CAD build for the part. Positions are in the model's coordinates, mm. Give positions to 0.01 mm unless a question says otherwise; leave off trailing zeros. Order: outer loops, then holes, each group sorted by start corner. A loop starts at its lowest first (then second) coordinate and runs counter-clockwise, first axis right, second up.
Autodesk Inventor part; units mm, degrees
ref_plane "HW_B_1_XY" through (-30.5, 7, 0) normal (0, 1, 0) x (0, 0, -1)
ref_plane "HW_B_1_YZ" through (-30.5, 7, 0) normal (0, 0, -1) x (-1, 0, 0)
ref_plane "HW_B_1_ZX" through (-30.5, 7, 0) normal (-1, 0, 0) x (0, 1, 0)
sketch "Sketch_1" plane through (0, 0, 0) normal (0, 0, 1) x (0, 1, 0)
  line L0 (3.8889, 0) -> (0, 0)
  arc A0 (0, 26.6) -> (0.6, 26) centre (0.6, 26.6) ccw
  line L1 (0.6, 26) -> (3.2889, 26)
  arc A1 (3.2889, 26) -> (3.8889, 26.6) centre (3.2889, 26.6) ccw
  line L2 (3.8889, 26.6) -> (3.8889, 28.8966)
  arc A2 (3.8889, 32.1034) -> (3.8889, 28.8966) centre (7, 30.5) ccw
  line L3 (3.8889, 32.1034) -> (3.8889, 34.4)
  arc A3 (3.8889, 34.4) -> (3.2889, 35) centre (3.2889, 34.4) ccw
  line L4 (3.2889, 35) -> (0.6, 35)
  arc A4 (0.6, 35) -> (0, 34.4) centre (0.6, 34.4) ccw
  line L5 (0, 34.4) -> (0, 26.6)
revolve "Revolution1" add sketch "Sketch_1" angle 360 about axis through (0, 3.8889, 0) along (0, 1, 0)
ref_plane "HW_B_1_XY" through (-30.5, 7, 0) normal (0, 1, 0) x (0, 0, -1)
ref_plane "HW_B_1_YZ" through (-30.5, 7, 0) normal (0, 0, -1) x (-1, 0, 0)
ref_plane "HW_B_1_ZX" through (-30.5, 7, 0) normal (-1, 0, 0) x (0, 1, 0)
ref_plane "HW_B_10_XY" through (30.5, 7, 0) normal (0, 1, 0) x (0, 0, -1)
ref_plane "HW_B_10_YZ" through (30.5, 7, 0) normal (0, 0, -1) x (-1, 0, 0)
ref_plane "HW_B_10_ZX" through (30.5, 7, 0) normal (-1, 0, 0) x (0, 1, 0)
ref_plane "HW_B_11_XY" through (28.6606, 7, -10.4316) normal (0, 1, 0) x (0, 0, -1)
ref_plane "HW_B_11_YZ" through (28.6606, 7, -10.4316) normal (0, 0, -1) x (-1, 0, 0)
ref_plane "HW_B_11_ZX" through (28.6606, 7, -10.4316) normal (-1, 0, 0) x (0, 1, 0)
ref_plane "HW_B_12_XY" through (23.3644, 7, -19.605) normal (0, 1, 0) x (0, 0, -1)
ref_plane "HW_B_12_YZ" through (23.3644, 7, -19.605) normal (0, 0, -1) x (-1, 0, 0)
ref_plane "HW_B_12_ZX" through (23.3644, 7, -19.605) normal (-1, 0, 0) x (0, 1, 0)
ref_plane "HW_B_13_XY" through (15.25, 7, -26.4138) normal (0, 1, 0) x (0, 0, -1)
ref_plane "HW_B_13_YZ" through (15.25, 7, -26.4138) normal (0, 0, -1) x (-1, 0, 0)
ref_plane "HW_B_13_ZX" through (15.25, 7, -26.4138) normal (-1, 0, 0) x (0, 1, 0)
ref_plane "HW_B_14_XY" through (5.2963, 7, -30.0366) normal (0, 1, 0) x (0, 0, -1)
ref_plane "HW_B_14_YZ" through (5.2963, 7, -30.0366) normal (0, 0, -1) x (-1, 0, 0)
ref_plane "HW_B_14_ZX" through (5.2963, 7, -30.0366) normal (-1, 0, 0) x (0, 1, 0)
ref_plane "HW_B_15_XY" through (-5.2963, 7, -30.0366) normal (0, 1, 0) x (0, 0, -1)
ref_plane "HW_B_15_YZ" through (-5.2963, 7, -30.0366) normal (0, 0, -1) x (-1, 0, 0)
ref_plane "HW_B_15_ZX" through (-5.2963, 7, -30.0366) normal (-1, 0, 0) x (0, 1, 0)
ref_plane "HW_B_16_XY" through (-15.25, 7, -26.4138) normal (0, 1, 0) x (0, 0, -1)
ref_plane "HW_B_16_YZ" through (-15.25, 7, -26.4138) normal (0, 0, -1) x (-1, 0, 0)
ref_plane "HW_B_16_ZX" through (-15.25, 7, -26.4138) normal (-1, 0, 0) x (0, 1, 0)
ref_plane "HW_B_17_XY" through (-23.3644, 7, -19.605) normal (0, 1, 0) x (0, 0, -1)
ref_plane "HW_B_17_YZ" through (-23.3644, 7, -19.605) normal (0, 0, -1) x (-1, 0, 0)
ref_plane "HW_B_17_ZX" through (-23.3644, 7, -19.605) normal (-1, 0, 0) x (0, 1, 0)
ref_plane "HW_B_18_XY" through (-28.6606, 7, -10.4316) normal (0, 1, 0) x (0, 0, -1)
ref_plane "HW_B_18_YZ" through (-28.6606, 7, -10.4316) normal (0, 0, -1) x (-1, 0, 0)
ref_plane "HW_B_18_ZX" through (-28.6606, 7, -10.4316) normal (-1, 0, 0) x (0, 1, 0)
ref_plane "HW_B_2_XY" through (-28.6606, 7, 10.4316) normal (0, 1, 0) x (0, 0, -1)
ref_plane "HW_B_2_YZ" through (-28.6606, 7, 10.4316) normal (0, 0, -1) x (-1, 0, 0)
ref_plane "HW_B_2_ZX" through (-28.6606, 7, 10.4316) normal (-1, 0, 0) x (0, 1, 0)
ref_plane "HW_B_3_XY" through (-23.3644, 7, 19.605) normal (0, 1, 0) x (0, 0, -1)
ref_plane "HW_B_3_YZ" through (-23.3644, 7, 19.605) normal (0, 0, -1) x (-1, 0, 0)
ref_plane "HW_B_3_ZX" through (-23.3644, 7, 19.605) normal (-1, 0, 0) x (0, 1, 0)
ref_plane "HW_B_4_XY" through (-15.25, 7, 26.4138) normal (0, 1, 0) x (0, 0, -1)
ref_plane "HW_B_4_YZ" through (-15.25, 7, 26.4138) normal (0, 0, -1) x (-1, 0, 0)
ref_plane "HW_B_4_ZX" through (-15.25, 7, 26.4138) normal (-1, 0, 0) x (0, 1, 0)
ref_plane "HW_B_5_XY" through (-5.2963, 7, 30.0366) normal (0, 1, 0) x (0, 0, -1)
ref_plane "HW_B_5_YZ" through (-5.2963, 7, 30.0366) normal (0, 0, -1) x (-1, 0, 0)
ref_plane "HW_B_5_ZX" through (-5.2963, 7, 30.0366) normal (-1, 0, 0) x (0, 1, 0)
ref_plane "HW_B_6_XY" through (5.2963, 7, 30.0366) normal (0, 1, 0) x (0, 0, -1)
ref_plane "HW_B_6_YZ" through (5.2963, 7, 30.0366) normal (0, 0, -1) x (-1, 0, 0)
ref_plane "HW_B_6_ZX" through (5.2963, 7, 30.0366) normal (-1, 0, 0) x (0, 1, 0)
ref_plane "HW_B_7_XY" through (15.25, 7, 26.4138) normal (0, 1, 0) x (0, 0, -1)
ref_plane "HW_B_7_YZ" through (15.25, 7, 26.4138) normal (0, 0, -1) x (-1, 0, 0)
ref_plane "HW_B_7_ZX" through (15.25, 7, 26.4138) normal (-1, 0, 0) x (0, 1, 0)
ref_plane "HW_B_8_XY" through (23.3644, 7, 19.605) normal (0, 1, 0) x (0, 0, -1)
ref_plane "HW_B_8_YZ" through (23.3644, 7, 19.605) normal (0, 0, -1) x (-1, 0, 0)
ref_plane "HW_B_8_ZX" through (23.3644, 7, 19.605) normal (-1, 0, 0) x (0, 1, 0)
ref_plane "HW_B_9_XY" through (28.6606, 7, 10.4316) normal (0, 1, 0) x (0, 0, -1)
ref_plane "HW_B_9_YZ" through (28.6606, 7, 10.4316) normal (0, 0, -1) x (-1, 0, 0)
ref_plane "HW_B_9_ZX" through (28.6606, 7, 10.4316) normal (-1, 0, 0) x (0, 1, 0)
ref_plane "HW_SW_XY" through (0, 0, 0) normal (0, 1, 0) x (0, 0, -1)
ref_plane "HW_SW_YZ" through (0, 0, 0) normal (0, 0, -1) x (-1, 0, 0)
ref_plane "HW_SW_ZX" through (0, 0, 0) normal (-1, 0, 0) x (0, 1, 0)
properties part number "51110 Housing washer"
1. Saw through at A-A on z = 0. Give the cut face in (x, y).
2. Mould opens along X. For faces 1 (the cylindrical face through (28, 2, 21)), 2 (the flat face through (-18, 0, -20)), 3 (the cylindrical face through (20.633, 1.963, -15.821)) say: released by +X, released by -X, zero draft, split by the parting line, or undercut.
3. Wall check: line 1 (Z direction, x = 0, y = 1.95); line 2 (X direction, y = 2.05, z = 9); line 3 (X direction, y = 2.1, z = -12). Give the ranges that are in metal, low to high.
4. Saw through at B-B on x = 0. Give the cut face in (y, z), plus the area to 3 significant figures.
5. Pin check, flat tip, straight feed: P1, Ø2, axis at y = 2.5, z = -4, coming from the +X side. Stop position of the tip, or through.
6. Saw through at C-C on y = 2. Give the cut face in (x, z).
Reported:
1. outline: (-35, 0.6) arc R0.6 ccw to (-34.4, 0) - (-26.6, 0) arc R0.6 ccw to (-26, 0.6) - (-26, 3.29) arc R0.6 ccw to (-26.6, 3.89) - (-28.9, 3.89) arc R3.5 cw to (-32.1, 3.89) - (-34.4, 3.89) arc R0.6 ccw to (-35, 3.29) - close; (26, 0.6) arc R0.6 ccw to (26.6, 0) - (34.4, 0) arc R0.6 ccw to (35, 0.6) - (35, 3.29) arc R0.6 ccw to (34.4, 3.89) - (32.1, 3.89) arc R3.5 cw to (28.9, 3.89) - (26.6, 3.89) arc R0.6 ccw to (26, 3.29) - close
2. face 1: split by the parting line
2. face 2: zero draft
2. face 3: undercut
3. line 1: z = -35 to -26, 26 to 35
3. line 2: x = -33.82 to -24.39, 24.39 to 33.82
3. line 3: x = -32.88 to -23.07, 23.07 to 32.88
4. outline: (0, -34.4) arc R0.6 ccw to (0.6, -35) - (3.29, -35) arc R0.6 ccw to (3.89, -34.4) - (3.89, -32.1) arc R3.5 cw to (3.89, -28.9) - (3.89, -26.6) arc R0.6 ccw to (3.29, -26) - (0.6, -26) arc R0.6 ccw to (0, -26.6) - close; (0, 26.6) arc R0.6 ccw to (0.6, 26) - (3.29, 26) arc R0.6 ccw to (3.89, 26.6) - (3.89, 28.9) arc R3.5 cw to (3.89, 32.1) - (3.89, 34.4) arc R0.6 ccw to (3.29, 35) - (0.6, 35) arc R0.6 ccw to (0, 34.4) - close
4. area: 67.7 mm2
5. P1: stops at x = 34.87
6. outline: circle Ø70 at (0, 0); hole circle Ø52 at (0, 0)
